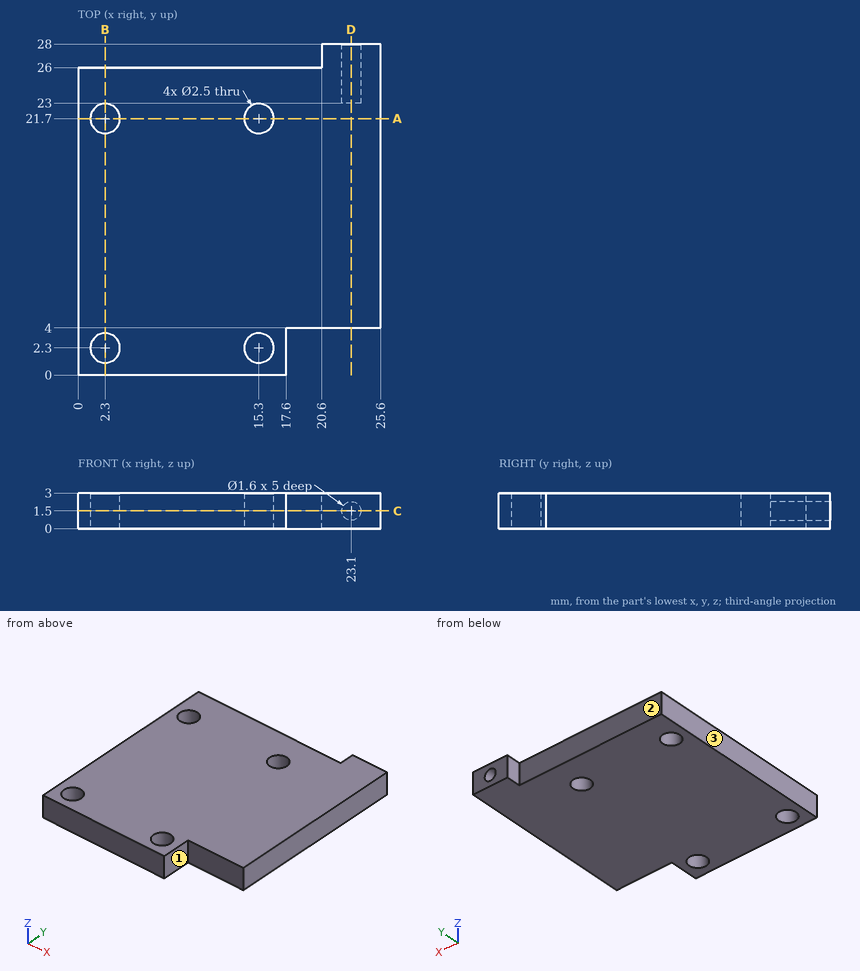
Part print with two shaded views. Sizes in mm from the minimum x, y, z corner. A direction names the side the tool comes from. Coordinates: 2 decimals unless noted, no trailing zeros. Write each loop counter-clockwise with the first axis right and the second up, starting at its lowest first coordinate (ties: lowest second). Pieces come first, ordered by that corner, then holes. Notation, with made-up numbers: (32.5, 11.25) - (60.5, 11.25) arc R8 ccw to (60.5, 26.25) - close; hole circle Ø9 at (-33.5, 86.25). An arc over 180 degrees is marked (long way). Put each result on its own line as item: value.
1. Flat gauge pins, fed straight in: pin 1 Ø1.3 at (x, z) = (23.5, 1) entering from +Y; pin 2 Ø1.5 at (x, z) = (21.5, 1.5) entering from -Y; pin 3 Ø0.6 at (y, z) = (27, 1) entering from -X. Where does each tip first touch, or does it go through?
Final values:
pin 1: stops at y = 28
pin 2: stops at y = 4
pin 3: stops at x = 20.6
2. Band-saw the part on B-B (x = 2.3). Write the cut outline in (y, z), then the cut area to 3 significant figures.
Final values:
outline: (0, 0) - (1.05, 0) - (1.05, 3) - (0, 3) - close; (3.55, 0) - (20.45, 0) - (20.45, 3) - (3.55, 3) - close; (22.95, 0) - (26, 0) - (26, 3) - (22.95, 3) - close
area: 63.0 mm²
3. Probe line 1 along Y through (x, z) = (15.3, 2.25); line 2 along Y through (x, z) = (14.75, 0.75); line 3 along X through (y, z) = (25.2, 1.5). List the from-to ranges inside material, lowest first. Write a range as [from, to].
Final values:
line 1: y = [0, 1.05], [3.55, 20.45], [22.95, 26]
line 2: y = [0, 1.18], [3.42, 20.58], [22.82, 26]
line 3: x = [0, 22.3], [23.9, 25.6]
4. 3-axis set-ups, long thin cutter, end or side, ignore diameter. For the marked faces 1, 2 and 3: which of +Z, -Z, +X, -X, +Y, -Y reach the whole face in a straight line?
Final values:
face 1: +Z, -Z, +X, -Y
face 2: +Z, -Z, -X, +Y
face 3: +Z, -Z, -X, +Y, -Y
5. Band-saw the part on A-A (y = 21.7). Write the cut outline in (x, z), then the cut area to 3 significant figures.
Final values:
outline: (0, 0) - (1.05, 0) - (1.05, 3) - (0, 3) - close; (3.55, 0) - (14.05, 0) - (14.05, 3) - (3.55, 3) - close; (16.55, 0) - (25.6, 0) - (25.6, 3) - (16.55, 3) - close
area: 61.8 mm²
6. Band-saw the part on D-D (x = 23.1). Write the cut outline in (y, z).
Final values:
outline: (4, 0) - (28, 0) - (28, 0.7) - (23, 0.7) - (23, 2.3) - (28, 2.3) - (28, 3) - (4, 3) - close
7. Band-saw the part on C-C (z = 1.5). Write the cut outline in (x, y), then the cut area to 3 significant figures.
Final values:
outline: (0, 0) - (17.6, 0) - (17.6, 4) - (25.6, 4) - (25.6, 28) - (23.9, 28) - (23.9, 23) - (22.3, 23) - (22.3, 28) - (20.6, 28) - (20.6, 26) - (0, 26) - close; hole circle Ø2.5 at (2.3, 2.3); hole circle Ø2.5 at (2.3, 21.7); hole circle Ø2.5 at (15.3, 2.3); hole circle Ø2.5 at (15.3, 21.7)
area: 616 mm²
